Autodesk Inventor part; units mm, degrees
ref_plane "YZ Plane" through (0, 0, 0) normal (1, 0, 0) x (0, 1, 0)
ref_plane "XZ Plane" through (0, 0, 0) normal (0, 1, 0) x (-1, 0, 0)
ref_plane "XY Plane" through (0, 0, 0) normal (0, 0, 1) x (1, 0, 0)
sketch "Boceto2" plane through (0, 0, 0) normal (1, 0, 0) x (0, 1, 0)
  circle A0 centre (0, 0) radius 4
  dimension "d3" = 8
extrude "Extrusión2" add sketch "Boceto2" along normal blind 19.5
sketch "Boceto3" plane through (0, 0, 0) normal (-1, 0, 0) x (0, 0, 1)
  circle A0 centre (0, 0) radius 4
  line L0 (-2.5, -5) -> (-2.5, 5)
  line L1 (-2.5, 5) -> (2.5, 5)
  line L2 (2.5, 5) -> (2.5, -5)
  line L3 (2.5, -5) -> (-2.5, -5)
  line L4 (-2.5, -5) -> (2.5, 5) construction
  line L5 (-2.5, 5) -> (2.5, -5) construction
  point P0 (-3.1225, 2.5)
  point P1 (-3.1225, -2.5)
  dimension "d15" = 10
  dimension "d16" = 5
extrude "Extrusión3" add sketch "Boceto3" against normal blind 9
sketch "Boceto4" plane through (0, 0, 0) normal (-1, 0, 0) x (0, 0, 1)
  line L0 (2.5, 3.1225) -> (2.5, -3.1225)
  line L1 (-2.5, 3.1225) -> (-2.5, -3.1225)
  line L2 (2.5, 5) -> (2.5, 3.1225)
  line L3 (-2.5, 3.1225) -> (-2.5, 5)
  arc A0 (2.5, -3.1225) -> (2.5, 3.1225) centre (0, 0) ccw
  arc A1 (-2.5, 3.1225) -> (-2.5, -3.1225) centre (0, 0) ccw
sketch "Boceto5" plane through (0, 0, 0) normal (-1, 0, 0) x (0, 0, 1)
  point P0 (0, 0)
extrude "Extrusión4" cut sketch "Boceto4" against normal blind 7
properties part number "Union pie"
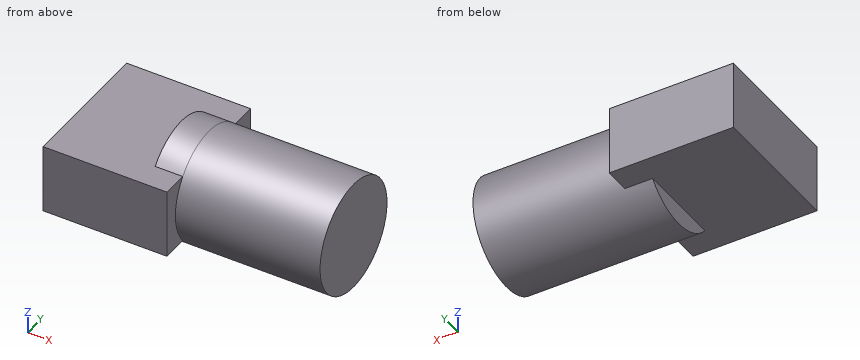
Could you check a few things on this model? Use its own coordinates, in mm. Give positions to 0.01 mm unless a question says otherwise; leave off trailing zeros. Order: outer loops, then holes, each group sorted by start corner. A loop starts at its lowest first (then second) coordinate and runs counter-clockwise, first axis right, second up. Notation, with made-up numbers: (60, 22.5) - (78, 22.5) arc R14 ccw to (78, 49.5) - close; hole circle Ø9 at (47, 59.25). An arc over 180 degrees is marked (long way). One line per item, written item: value. Start each with the question number.
1. For P1, Ø0.5, axis at y = 1, z = -3, coming from the -X side, with a flat end and sliding along its axis, tell me the tip position at first contact or that it passes through.
2. Imagine slicing it at A-A on z = 0. List the corners of the cut face in (x, y) for me.
3. If I drill on probe 1 along X at (y, z) = (-1, -3); probe 2 along Z at (x, y) = (5, 2); probe 3 along Z at (x, y) = (8.25, -3), over which ranges is the centre line in solid material (lowest first)?
4. Imagine slicing it at B-B on y = 0. List the corners of the cut face in (x, z) for me, plus the area to 3 significant figures.
5. Imagine slicing it at D-D on x = 16.25. List the corners of the cut face in (y, z) for me, plus the area to 3 significant figures.
6. Imagine slicing it at C-C on x = 4.5. List the corners of the cut face in (y, z) for me.
Values:
1. P1: x = 7
2. outline: (0, -5) - (9, -5) - (9, -4) - (19.5, -4) - (19.5, 4) - (9, 4) - (9, 5) - (0, 5) - close
3. probe 1: 7 to 19.5
3. probe 2: -2.5 to 2.5
3. probe 3: -2.65 to 2.65
4. outline: (0, -2.5) - (7, -2.5) - (7, -4) - (19.5, -4) - (19.5, 4) - (7, 4) - (7, 2.5) - (0, 2.5) - close
4. area: 135 mm²
5. outline: circle Ø8 at (0, 0)
5. area: 50.3 mm²
6. outline: (-5, -2.5) - (5, -2.5) - (5, 2.5) - (-5, 2.5) - close
